Verification items for the finished model (mm, model axes). A direction names the side the tool comes from. Give positions to 0.01 mm unless a question says otherwise; leave off trailing zeros. Loops run counter-clockwise (first coordinate to the right, second up) from the corner with the lowest first, then second, coordinate; pieces in that order, holes last. Notation, with made-up numbers: (48.5, -20.5) -> (58.5, -20.5) arc R34 cw to (58.5, 9.5) -> close; hole circle Ø1 at (-2, 32.5). An arc over 180 degrees is marked (long way). Use one line per item in the form item = value. Start each with the question number.
Autodesk Inventor part; units mm, degrees
ref_plane "YZ Plane" through (0, 0, 0) normal (1, 0, 0) x (0, 1, 0)
ref_plane "XZ Plane" through (0, 0, 0) normal (0, 1, 0) x (-1, 0, 0)
ref_plane "XY Plane" through (0, 0, 0) normal (0, 0, 1) x (1, 0, 0)
sketch "草圖1" plane through (0, 0, 0) normal (0, 1, 0) x (-1, 0, 0)
  line L0 (0, 0) -> (6, 0)
  line L1 (6, 0) -> (6, -70)
  line L2 (6, -70) -> (0, -70)
  line L3 (0, -70) -> (0, 0)
  line L4 (0, 0) -> (6, 0)
  line L5 (6, 0) -> (6, 3)
  line L6 (6, 3) -> (0, 3)
  line L7 (0, 3) -> (0, 0)
  line L8 (6, 0) -> (18, -67)
  line L9 (18, -67) -> (18, -70)
  line L10 (18, -70) -> (6, -70)
  circle A0 centre (1.5, 1.5) radius 0.25
  circle A1 centre (3, -12) radius 0.25
  point P0 (6, 1.5)
  dimension "d0" = 70
  dimension "d1" = 6
  dimension "d2" = 3
  dimension "d5" = 12
  dimension "d6" = 3
  dimension "d7" = 0.5
  dimension "d8" = 0.5
  dimension "d9" = 15
  dimension "d10" = 3
extrude "擠出1" add sketch "草圖1" along normal blind 3
Item 1: Sectioned sample at C-C, the plane x = -9.5. Enter the section's corners in (y, z).
Item 2: Sectioned sample at A-A, the plane y = 0.55. Enter the section's corners in (x, z).
Item 3: Tool access check on faces 1 (the flat face through (-7, 3, -41)), 2 (the flat face through (-6, 1, 1)). Record the directions out of +Z, -Z, +X, -X, +Y, -Y that give a thin tool (end or side, any length) a straight path to the whole face; none if there is none.
Item 4: Gauge pin test, flat ends, axial feed: pin 1 Ø0.9 at (y, z) = (1, 2) entering from -X; pin 2 Ø1.5 at (y, z) = (1, -10.5) entering from -X. Record the tip position at first contact, or that the pin passes through.
Item 5: Sectioned sample at B-B, the plane z = -43. Enter the section's corners in (x, y), and give its area (3 significant figures).
Item 6: Material ranges on line 1 (Z direction, x = -1.5, y = 0.8); line 2 (Z direction, x = -3, y = 0.85); line 3 (X direction, y = 1.4, z = -5), recorded low to high.
Outcome:
q1.outline = (0, -70) -> (3, -70) -> (3, -19.54) -> (0, -19.54) -> close
q2.outline = (-18, -70) -> (0, -70) -> (0, 3) -> (-6, 3) -> (-6, 0) -> (-18, -67) -> close; hole circle Ø0.5 at (-3, -12); hole circle Ø0.5 at (-1.5, 1.5)
q3.face_1 = +Z, -Z, +X, -X, +Y
q3.face_2 = +Z, -X, +Y, -Y
q4.pin_1 = -6
q4.pin_2 = -8.01
q5.outline = (-13.7, 0) -> (0, 0) -> (0, 3) -> (-13.7, 3) -> close
q5.area = 41.1 mm^2
q6.line_1 = -70 to 1.25, 1.75 to 3
q6.line_2 = -70 to -12.25, -11.75 to 3
q6.line_3 = -6.9 to 0
